Here's how the part is built. I have some questions about the finished solid (model axes, mm). Round coordinates to 2 decimals unless told otherwise and drop trailing zeros. Write each loop counter-clockwise with the first axis right and the second up, starting at its lowest first coordinate (ties: lowest second). Pieces come first, ordered by that corner, then holes. Notation, with made-up numbers: (1, -8.5) - (43, -8.5) arc R10 ccw to (43, 10.5) - close; hole circle Ø4 at (83.5, 81.25). An arc over 180 degrees is marked (long way). Write item = value, one per line. Start each with the question number.
Item 1: If I drill on line 1 along Z through (x, y) = (46.5, 1.55); line 2 along X through (y, z) = (2.25, 90); line 3 along Z through (x, y) = (16, 1.3), over which ranges is the centre line in solid material (lowest first)? Write a range as [from, to].
Item 2: If we section it at C-C (x = 32.5): Please give me the cut outline in (y, z), and give its area (3 significant figures).
Item 3: If we section it at A-A (z = 52.5): Please give me the cut outline in (x, y), and give its area (3 significant figures).
Item 4: For P1, Ø0.9, axis at y = 2, z = 9, coming from the +X side; P2, Ø1.5, axis at y = 2, z = 46, coming from the -X side; P3, Ø1.5, axis at x = 47.5, y = 2, coming from the +Z side, each with a flat end and sliding along its axis, tell me the tip position at first contact or that it passes through.
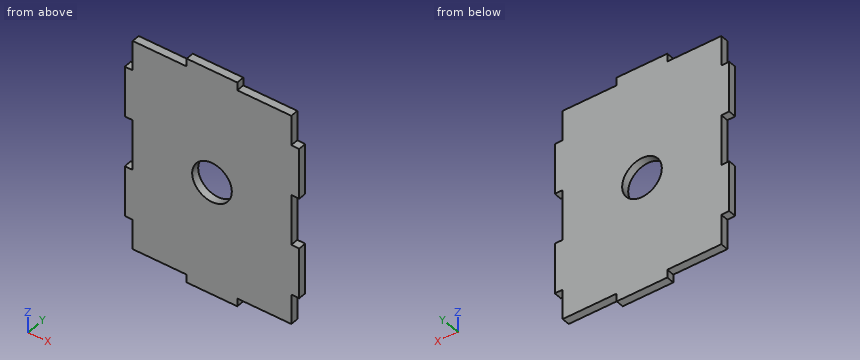
```python
from build123d import *

# Parameters (mm, degrees)
SKETCH1_R           = 7.5
BOSS_EXTRUDE1_DEPTH = 3


with BuildPart() as part:
    # Sketch1 → Boss-Extrude1 (new body)
    with BuildSketch(Plane(origin=(0, 0, 0), x_dir=(1, 0, 0), z_dir=(0, 1, 0))):
        Polygon((-13.885581934, -10.773206129), (-13.885581934, -22.085706129), (-16.885581934, -22.085706129), (-16.885581934, -41.210706129), (-13.885581934, -41.210706129), (-13.885581934, -60.335706129), (-16.885581934, -60.335706129), (-16.885581934, -79.460706129), (-13.885581934, -79.460706129), (-13.885581934, -90.773206129), (6.551918066, -90.773206129), (6.551918066, -93.773206129), (25.676918066, -93.773206129), (25.676918066, -90.773206129), (44.801918066, -90.773206129), (46.114418066, -90.773206129), (46.114418066, -79.460706129), (49.114418066, -79.460706129), (49.114418066, -60.335706129), (46.114418066, -60.335706129), (46.114418066, -41.210706129), (49.114418066, -41.210706129), (49.114418066, -22.085706129), (46.114418066, -22.085706129), (46.114418066, -10.773206129), (25.676918066, -10.773206129), (25.676918066, -7.773206129), (6.551918066, -7.773206129), (6.551918066, -10.773206129), (-12.573081934, -10.773206129), align=None)
        with Locations(Location((16.114418066, -50.773206129, 0), (0, 0, 270))):
            Circle(SKETCH1_R, mode=Mode.SUBTRACT)
    extrude(amount=BOSS_EXTRUDE1_DEPTH)


solid = part.part
```
Reply:
q1.line_1 = [22.09, 41.21], [60.34, 79.46]
q1.line_2 = [-13.89, 46.11]
q1.line_3 = [7.77, 43.27], [58.27, 93.77]
q2.outline = (0, 10.77) - (3, 10.77) - (3, 90.77) - (0, 90.77) - close
q2.area = 240 mm2
q3.outline = (-13.89, 0) - (8.82, 0) - (8.82, 3) - (-13.89, 3) - close; (23.41, 0) - (46.11, 0) - (46.11, 3) - (23.41, 3) - close
q3.area = 136 mm2
q4.P1 = 25.68
q4.P2 = -13.89
q4.P3 = 79.46
